The model under review builds one solid part; all positions refer to its coordinate system, in mm. Face numbers are marked on the shaded views. A direction names the side the tool comes from. Give positions to 0.01 mm unless a question says otherwise; leave off trailing zeros. Loops run counter-clockwise (first coordinate to the right, second up) from the corner with the lowest first, then second, coordinate; pieces in that order, holes last. Notation, with made-up numbers: (43, -17.75) -> (93, -17.75) arc R31 ccw to (93, 7.25) -> close; hole circle Ø5 at (-21.5, -29). An arc over 180 degrees is marked (long way). Write each question's results on one line, items separated by ' | '. Start each with the question number.
Q1. We need section C-C (x = 24.5). Write out the cut boundary in (y, z), plus the area to 3 significant figures.
Q2. Wall thickness on L1, parallel to X at y = 5.5, z = -4.5; L2, parallel to Y at x = 25.5, z = -2.5; L3, parallel to Y at x = 21.25, z = 3.5: over which ranges is each line inside the solid? List them lowest first. Write a range as [from, to].
Q3. Machinability: for the marked faces 1 and 2, which of the approach directions +Z, -Z, +X, -X, +Y, -Y give a long, thin tool a straight path to every point of the face, cutting with its end or side? Answer none if there is none.
Q4. We need section A-A (z = 0). Write out the cut boundary in (x, y).
from build123d import *

# Parameters (mm, degrees)
SKETCH1_W           = 12.7
SKETCH1_H           = 12.7
BOSS_EXTRUDE1_DEPTH = 12
SKETCH2_R           = 4
BOSS_EXTRUDE2_DEPTH = 16
FILLET1_R           = 0.5
CHAMFER2_SIZE       = 0.5


with BuildPart() as part:
    # Sketch1 → Boss-Extrude1 (new body)
    with BuildSketch(Plane(origin=(0, 0, 0), x_dir=(0, 0, -1), z_dir=(1, 0, 0))):
        Rectangle(SKETCH1_W, SKETCH1_H)
    extrude(amount=BOSS_EXTRUDE1_DEPTH)

    # Sketch2 → Boss-Extrude2 (add)
    with BuildSketch(Plane(origin=(12, 0, 0), x_dir=(0, 0, -1), z_dir=(1, 0, 0))):
        Circle(SKETCH2_R)
    extrude(amount=BOSS_EXTRUDE2_DEPTH)

    # Fillet1
    fillet1_edges = [part.edges().sort_by_distance(p)[0] for p in [
        (12, 0, 4),
    ]]
    fillet(fillet1_edges, radius=FILLET1_R)

    # Chamfer2
    chamfer2_edges = [part.edges().sort_by_distance(p)[0] for p in [
        (0, 6.35, 0),
        (0, 0, -6.35),
        (0, -6.35, 0),
        (0, 0, 6.35),
    ]]
    chamfer(chamfer2_edges, length=CHAMFER2_SIZE)


solid = part.part
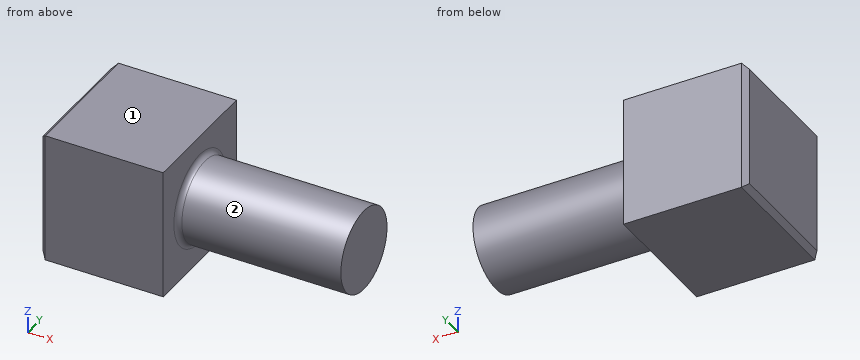
Output:
1) outline: circle Ø8 at (0, 0) | area: 50.3 mm2
2) L1: [0, 12] | L2: [-3.12, 3.12] | L3: [-1.94, 1.94]
3) face 1: +Z, +X, -X, +Y, -Y | face 2: +X
4) outline: (0, -5.85) -> (0.5, -6.35) -> (12, -6.35) -> (12, -4.5) arc R0.5 cw to (12.5, -4) -> (28, -4) -> (28, 4) -> (12.5, 4) arc R0.5 cw to (12, 4.5) -> (12, 6.35) -> (0.5, 6.35) -> (0, 5.85) -> close
